Could you check a few things on this model? Use its own coordinates, in mm. A direction names the side the tool comes from. Coordinates: 2 decimals unless noted, no trailing zeros. Order: outer loops, then holes, each group sorted by start corner. A loop starts at its lowest first (then second) coordinate and runs counter-clockwise, first axis right, second up. Notation, with made-up numbers: (37, 30.25) -> (70, 30.25) arc R6 ccw to (70, 35.25) -> close; hole circle Ø2 at (85.25, -21.5). An arc over 180 degrees is marked (long way). Use a Markdown table: item, result. Add a question column.
1) Thinking about a two-plate mould opening in X: for faces 1 (the cylindrical face through (0, -15, 11)), 2 (the cylindrical face through (6.794, 4.949, 5.479)), 3 (the flat face through (10, 0, 1)), which applies, +X half, -X half, draft (parallel to the pull), parting line (faces both ways), or undercut?
2) Which directions (+Z, -Z, +X, -X, +Y, -Y) give clear straight access to the entire face, cutting with the end or side of a thin tool? Please do faces 4 (the cylindrical face through (-5, 4.3, 5.5)), 5 (the flat face through (0, 0, 0)), 6 (the cylindrical face through (-0.074, 6.544, 2.986)).
3) If I drill on L1, parallel to X at y = -15.5, z = 13.5; L2, parallel to Z at x = -3.25, y = -5.5; L3, parallel to Z at x = -3.5, y = 1.5, over which ranges is the centre line in solid material (lowest first)? Write a range as [from, to].
4) If we section it at A-A (x = 6): Write out the boundary of the cut face in (y, z).
5) If we section it at B-B (z = 11): Write out the boundary of the cut face in (x, y), plus the area to 3 significant figures.
6) Will these pins go through, and if not, where does the flat tip stop? pin 1 Ø3 at (y, z) = (-8, 4.5) entering from +X; pin 2 Ø7.5 at (x, y) = (4, 3) entering from +Z; pin 3 Ø6 at (x, y) = (2.5, -13) entering from +Z.
7) If we section it at C-C (x = -8): Write out the boundary of the cut face in (y, z), plus the area to 3 significant figures.
8) If we section it at D-D (z = 13.5): Write out the boundary of the cut face in (x, y).
```python
from build123d import *

# Parameters (mm, degrees)
SKETCH1_W           = 20
SKETCH1_H           = 16
BOSS_EXTRUDE1_DEPTH = 2
BOSS_EXTRUDE2_DEPTH = 2
BOSS_EXTRUDE3_DEPTH = 1
FILLET1_START       = -2
FILLET1_DEPTH       = 4
SKETCH4_R           = 1
BOSS_EXTRUDE4_DEPTH = 3


with BuildPart() as part:
    # Sketch1 → Boss-Extrude1 (new body)
    with BuildSketch(Plane.XY):
        Rectangle(SKETCH1_W, SKETCH1_H)
    extrude(amount=BOSS_EXTRUDE1_DEPTH)

    # Sketch2 → Boss-Extrude2 (add)
    with BuildSketch(Plane.XY.offset(2)):
        with BuildLine():
            Line((-1, -8), (-1, -5.19120215))
            ThreePointArc((-1, -5.19120215), (-3.662465131, -1.222418993), (-7.438132905, 1.707477453))
            ThreePointArc((-7.438132905, 1.707477453), (-8.78383647, 5.458451445), (-5.217391304, 7.236425814))
            ThreePointArc((-5.217391304, 7.236425814), (0, 6.543906954), (5.217391304, 7.236425814))
            ThreePointArc((5.217391304, 7.236425814), (8.78383647, 5.458451445), (7.438132905, 1.707477453))
            ThreePointArc((7.438132905, 1.707477453), (3.662465131, -1.222418993), (1, -5.19120215))
            Line((1, -5.19120215), (1, -8))
            Line((1, -8), (-1, -8))
        make_face()
    extrude(amount=BOSS_EXTRUDE2_DEPTH)

    # Sketch3 → Boss-Extrude3 (add, symmetric)
    with BuildSketch(Plane(origin=(0, 0, 0), x_dir=(0, 0, -1), z_dir=(1, 0, 0))):
        with BuildLine():
            Line((-4, -8), (-2, -8))
            ThreePointArc((-2, -8), (-11, -17), (-20, -8))
            Line((-20, -8), (-18, -8))
            ThreePointArc((-18, -8), (-11, -15), (-4, -8))
        make_face()
    extrude(amount=BOSS_EXTRUDE3_DEPTH, both=True)

    # Fillet1: read off the stored shape, not the designer's step
    # Fillet1 outline → Fillet1 (cut)
    with BuildSketch(Plane.YZ.offset(FILLET1_START)):
        with BuildLine():
            ThreePointArc((-8, 20), (-8.563606213, 19.982335333), (-9.125, 19.929410675))
            add(Edge.make_bspline(
                [(-9.125, 19.929410675), (-8.857196429, 19.963150753), (-8.534549287, 19.913651104), (-8.211558936, 19.723387149), (-8.000000009, 19.372242351), (-8, 18.937253953)],
                knots=[0, 0, 0, 0, 0, 0, 0.531373028, 0.531373028, 0.531373028, 0.531373028, 0.531373028, 0.531373028], degree=5, weights=[1, 0.787450789, 0.631373036, 0.531766743, 0.488631909, 0.501968534]))
            Line((-8, 18.937253953), (-8, 20))
        make_face()
        with BuildLine():
            Line((-8, 18), (-8, 18.937253953))
            add(Edge.make_bspline(
                [(-8, 18.937253953), (-7.999999993, 18.572372269), (-8.153666641, 18.269213464), (-8.39236455, 18.072074091), (-8.646114708, 17.973934028), (-8.875, 17.945097192)],
                knots=[0.531373028, 0.531373028, 0.531373028, 0.531373028, 0.531373028, 0.531373028, 1, 1, 1, 1, 1, 1], degree=5, weights=[0.501968534, 0.513730332, 0.569414377, 0.66902067, 0.812549211, 1]))
            ThreePointArc((-8.875, 17.945097192), (-8.438360388, 17.986260815), (-8, 18))
        make_face()
    extrude(amount=FILLET1_DEPTH, mode=Mode.SUBTRACT)

    # Sketch4 → Boss-Extrude4 (add)
    with BuildSketch(Plane.XY.offset(4)):
        with Locations(Location((-6, 4.340303643, 0), (0, 0, 180))):
            Circle(SKETCH4_R)
        with Locations(Location((6, 4.340303643, 0), (0, 0, 180))):
            Circle(SKETCH4_R)
    extrude(amount=BOSS_EXTRUDE4_DEPTH)


solid = part.part
```
Answer sheet:
| question | item | result |
|---|---|---|
| 1 | face 1 | draft |
| 1 | face 2 | undercut |
| 1 | face 3 | +X half |
| 2 | face 4 | +Z |
| 2 | face 5 | -Z, +X, -X, +Y, -Y |
| 2 | face 6 | +Z, +Y |
| 3 | L1 | [-1, 1] |
| 3 | L2 | [0, 2] |
| 3 | L3 | [0, 4] |
| 4 | outline | (-8, 0) -> (8, 0) -> (8, 2) -> (7.34, 2) -> (7.34, 4) -> (5.34, 4) -> (5.34, 7) -> (3.34, 7) -> (3.34, 4) -> (0.81, 4) -> (0.81, 2) -> (-8, 2) -> close |
| 5 | outline | (-1, -17) -> (1, -17) -> (1, -15) -> (-1, -15) -> close |
| 5 | area | 4.00 mm2 |
| 6 | pin 1 | x = 1 |
| 6 | pin 2 | z = 7 |
| 6 | pin 3 | z = 19.67 |
| 7 | outline | (-8, 0) -> (8, 0) -> (8, 2) -> (6.58, 2) -> (6.58, 4) -> (2.1, 4) -> (2.1, 2) -> (-8, 2) -> close |
| 7 | area | 40.9 mm2 |
| 8 | outline | (-1, -16.65) -> (1, -16.65) -> (1, -14.54) -> (-1, -14.54) -> close |
